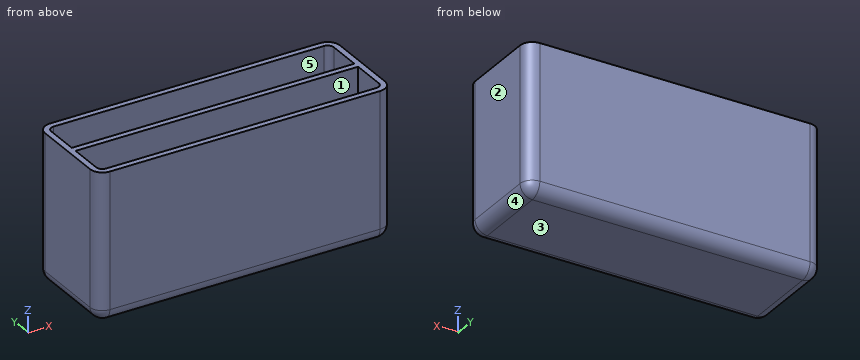
from build123d import *

# Parameters (mm, degrees)
SKETCH_W     = 1200
SKETCH_H     = 400
PAD_DEPTH    = 300
FILLET_R     = 50
THICKNESS_T  = -25
SKETCH001_W  = 1150
SKETCH001_H  = 25
PAD001_DEPTH = 575


with BuildPart() as part:
    # Sketch → Pad (new body, symmetric)
    with BuildSketch(Plane.XY):
        Rectangle(SKETCH_W, SKETCH_H)
    extrude(amount=PAD_DEPTH, both=True)

    # Fillet
    fillet_edges = [part.edges().sort_by_distance(p)[0] for p in [
        (600, 200, 0),
        (600, -200, 0),
        (-600, 0, -300),
        (0, -200, -300),
        (600, 0, -300),
        (0, 200, -300),
        (-600, -200, 0),
        (-600, 200, 0),
    ]]
    fillet(fillet_edges, radius=FILLET_R)

    # Thickness
    thickness_openings = [part.faces().sort_by_distance(p)[0] for p in [
        (0, 0, 300),
    ]]
    offset(amount=THICKNESS_T, openings=thickness_openings)

    # Sketch001 (on Face18 of Thickness) → Pad001 (join)
    with BuildSketch(Plane.XY.offset(300)):
        Rectangle(SKETCH001_W, SKETCH001_H)
    extrude(amount=-PAD001_DEPTH)


solid = part.part
Source: CAD feature listing. Evaluate the final solid. Frame: model axes, mm. Face numbers are marked on the shaded views. A direction names the side the tool comes from. Coordinates: 2 decimals unless noted, no trailing zeros. Loops run counter-clockwise (first coordinate to the right, second up) from the corner with the lowest first, then second, coordinate; pieces in that order, holes last. Notation, with made-up numbers: (-9, 15) - (34, 15) arc R17 ccw to (34, 24) - close; hole circle Ø9 at (0.5, -24). An arc over 180 degrees is marked (long way). One line per question, with ' | ' between items.
1) Set-up query: the marked faces 4 and 5. Return all of +Z, -Z, +X, -X, +Y, -Y with unobstructed straight access to the full face (end or side cutting, diameter ignored); none if empty.
Report:
face 4: -Z, +X, +Y, -Y | face 5: +Z
2) Line query: line 1 along Y through (x, z) = (25, 172); line 2 along X through (y, z) = (-66.5, -173); line 3 along Y through (x, z) = (-336.5, -260.5). Output: solid intervals per line, ascending.
Report:
line 1: y = -200 to -175, -12.5 to 12.5, 175 to 200 | line 2: x = -600 to -575, 575 to 600 | line 3: y = -198.89 to -172.69, -12.5 to 12.5, 172.69 to 198.89
3) Section B-B, the plane x = -6. Return loops of the section in (y, z).
Report:
outline: (-200, -250) arc R50 ccw to (-150, -300) - (150, -300) arc R50 ccw to (200, -250) - (200, 300) - (175, 300) - (175, -250) arc R25 cw to (150, -275) - (12.5, -275) - (12.5, 300) - (-12.5, 300) - (-12.5, -275) - (-150, -275) arc R25 cw to (-175, -250) - (-175, 300) - (-200, 300) - close
4) Section C-C, the plane y = -96. Return loops of the section in (x, z), then the cut area to 3 significant figures.
Report:
outline: (-600, -250) arc R50 ccw to (-550, -300) - (550, -300) arc R50 ccw to (600, -250) - (600, 300) - (575, 300) - (575, -250) arc R25 cw to (550, -275) - (-550, -275) arc R25 cw to (-575, -250) - (-575, 300) - (-600, 300) - close | area: 57,900 mm²
5) First-contact query: P1, Ø8, axis at x = -60, y = -120, coming from the +Z side. Flat tip, straight axial feed; report the tip coordinate or a pass-through.
Report:
P1: stops at z = -275
6) Pull-direction query (X, two-part tool) for the marked faces 1, 2 and 3; classes: released by +X, released by -X, zero draft, split by the parting line, or undercut.
Report:
face 1: undercut | face 2: released by +X | face 3: zero draft
7) Section A-A, the plane z = 186.5. Return loops of the section in (x, y).
Report:
outline: (-600, -150) arc R50 ccw to (-550, -200) - (550, -200) arc R50 ccw to (600, -150) - (600, 150) arc R50 ccw to (550, 200) - (-550, 200) arc R50 ccw to (-600, 150) - close; hole (-575, -150) arc R25 ccw to (-550, -175) - (550, -175) arc R25 ccw to (575, -150) - (575, -12.5) - (-575, -12.5) - close; hole (-575, 12.5) - (575, 12.5) - (575, 150) arc R25 ccw to (550, 175) - (-550, 175) arc R25 ccw to (-575, 150) - close
